from build123d import *

# Parameters (mm, degrees)
CROQUIS1_R              = 36.5
SALIENTE_EXTRUIR1_DEPTH = 38.4
CROQUIS2_R              = 39
SALIENTE_EXTRUIR2_DEPTH = 1.8
CROQUIS3_R              = 8.5
CORTAR_EXTRUIR1_DEPTH   = 43


with BuildPart() as part:
    # Croquis1 → Saliente-Extruir1 (new body)
    with BuildSketch(Plane.XY):
        Circle(CROQUIS1_R)
    extrude(amount=SALIENTE_EXTRUIR1_DEPTH)

    # Croquis2 → Saliente-Extruir2 (add)
    with BuildSketch(Plane.XY.offset(38.4)):
        Circle(CROQUIS2_R)
    saliente_extruir2 = extrude(amount=SALIENTE_EXTRUIR2_DEPTH)

    # Simetría1: Saliente-Extruir2 across plane
    add(saliente_extruir2.mirror(Plane(origin=(0, 0, 19.2), x_dir=(1, 0, 0), z_dir=(0, 0, -1))))

    # Croquis3 → Cortar-Extruir1 (cut, through all)
    with BuildSketch(Plane(origin=(0, 0, -1.8), x_dir=(-1, 0, 0), z_dir=(0, 0, -1))):
        Circle(CROQUIS3_R)
    extrude(amount=-CORTAR_EXTRUIR1_DEPTH, mode=Mode.SUBTRACT)


solid = part.part
Geometry: final body of the model. Coordinates: model frame, mm. A direction names the side the tool comes from. Give positions to 0.01 mm unless a question says otherwise; leave off trailing zeros. Loops run counter-clockwise (first coordinate to the right, second up) from the corner with the lowest first, then second, coordinate; pieces in that order, holes last. Notation, with made-up numbers: (68, 77.5) -> (75, 77.5) arc R11 ccw to (75, 97.5) -> close; hole circle Ø8 at (57.25, -23.5). An arc over 180 degrees is marked (long way). Put each result on its own line as item: value.
1. Cut plane C-C (y = -13). Return the cut outline in (x, z), plus the area to 3 significant figures.
Taken from the geometry:
outline: (-36.77, -1.8) -> (36.77, -1.8) -> (36.77, 0) -> (34.11, 0) -> (34.11, 38.4) -> (36.77, 38.4) -> (36.77, 40.2) -> (-36.77, 40.2) -> (-36.77, 38.4) -> (-34.11, 38.4) -> (-34.11, 0) -> (-36.77, 0) -> close
area: 2,880 mm2
2. Pull-direction query (X, two-part tool) for faces 3 (the cylindrical face through (-7.912, -35.632, 18.931)), 4 (the cylindrical face through (-4.57, 7.167, 18.906)), 5 (the flat face through (-1, 9, 40.2)); classes: released by +X, released by -X, zero draft, split by the parting line, or undercut.
Taken from the geometry:
face 3: split by the parting line
face 4: undercut
face 5: zero draft
3. Ray query, line 1 along Y through (x, z) = (0, 18.5); line 2 along Z through (x, y) = (30, 21); line 3 along X through (y, z) = (-7, 27.5). Return the intervals inside material, ascending. Write a range as [from, to].
Taken from the geometry:
line 1: y = [-36.5, -8.5], [8.5, 36.5]
line 2: z = [-1.8, 0], [38.4, 40.2]
line 3: x = [-35.82, -4.82], [4.82, 35.82]
4. Cut plane A-A (y = 0). Return the cut outline in (x, z).
Taken from the geometry:
outline: (-39, -1.8) -> (-8.5, -1.8) -> (-8.5, 40.2) -> (-39, 40.2) -> (-39, 38.4) -> (-36.5, 38.4) -> (-36.5, 0) -> (-39, 0) -> close; (8.5, -1.8) -> (39, -1.8) -> (39, 0) -> (36.5, 0) -> (36.5, 38.4) -> (39, 38.4) -> (39, 40.2) -> (8.5, 40.2) -> close
5. Cut plane D-D (z = 25.5). Return the cut outline in (x, y).
Taken from the geometry:
outline: circle Ø73 at (0, 0); hole circle Ø17 at (0, 0)
6. Set-up query: faces 1 (the cylindrical face through (-5.077, 38.668, 39.287)), 2 (the flat face through (26, -26, 38.4)). Return all of +Z, -Z, +X, -X, +Y, -Y with unobstructed straight access to the full face (end or side cutting, diameter ignored); none if empty.
Taken from the geometry:
face 1: +Z, -Z
face 2: none
7. Pin query (flat end, axial travel): P1, Ø13.5, axis at x = 0, y = 0, coming from the +Z side; P2, Ø4, axis at x = 23, z = 15, coming from the +Y side; P3, Ø8, axis at y = -20.5, z = 21, coming from the +X side; P4, Ø4, axis at x = -29.5, z = 26, coming from the -Y side. Return the tip coordinate at first contact, or that it passes through.
Taken from the geometry:
P1: passes through
P2: stops at y = 29.85
P3: stops at x = 32.56
P4: stops at y = -24
